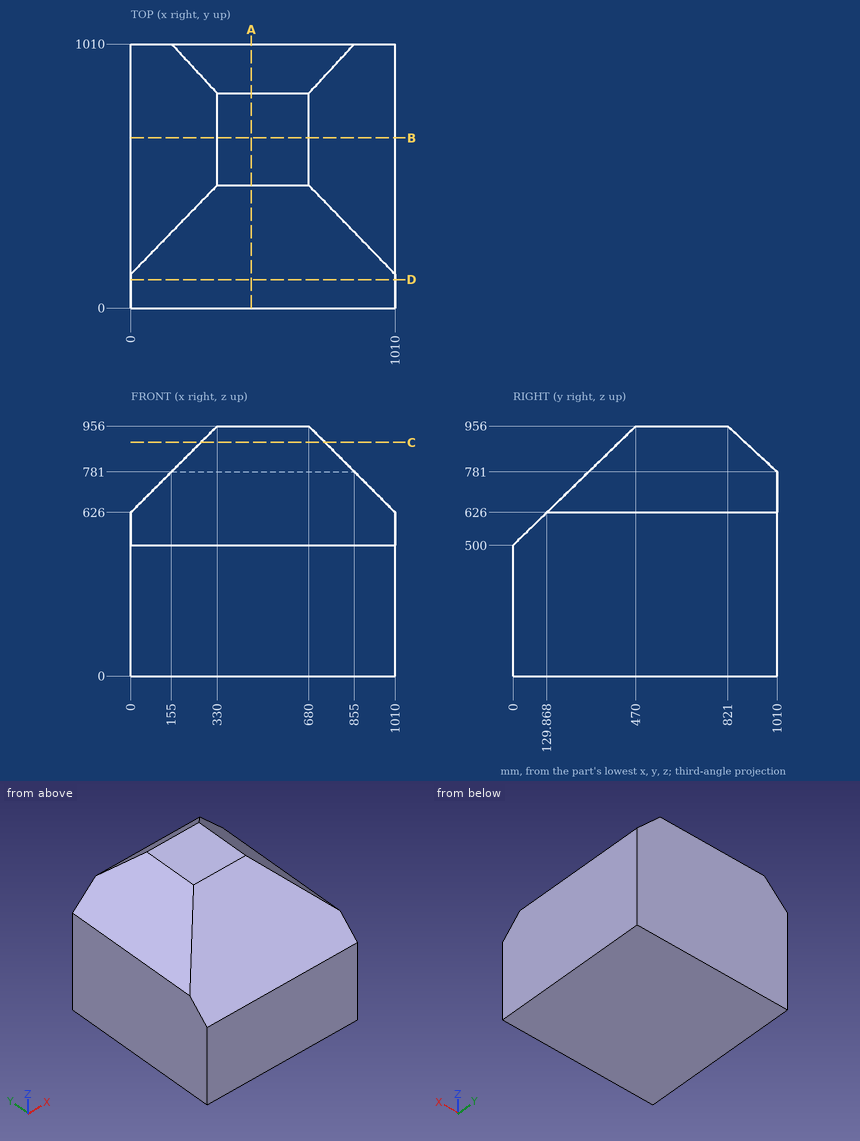
Study the drawing (mm; zero at the part's minimum x, y, z) and answer. Coordinates: 2 decimals unless noted, no trailing zeros. Write each loop counter-clockwise with the first axis right and the second up, starting at its lowest first coordinate (ties: lowest second). Pieces come first, ordered by that corner, then holes.
Q1. Section B-B, the plane y = 650.5 is taken. Write down the section's boundary in (x, z).
Returned:
outline: (0, 0) - (1010, 0) - (1010, 626) - (680, 956) - (330, 956) - (0, 626) - close
Q2. Section A-A, the plane x = 461 is taken. Write down the section's boundary in (y, z).
Returned:
outline: (0, 0) - (1010, 0) - (1010, 781) - (821, 956) - (470, 956) - (0, 500) - close
Q3. Find the intervals of material crossed by line 1 along X through (y, z) = (655.5, 748); line 2 along Z through (x, y) = (707, 577); line 3 along Y through (x, z) = (162, 761.5), in increasing order.
Returned:
line 1: x = 122 to 888
line 2: z = 0 to 929
line 3: y = 269.53 to 1010
Q4. Section C-C, the plane z = 893.5 is taken. Write down the section's boundary in (x, y).
Returned:
outline: (267.5, 405.58) - (742.5, 405.58) - (742.5, 888.5) - (267.5, 888.5) - close
Q5. Given P1, Ø5, axis at x = 594, z = 720, coming from the -Y side; P2, Ø6, axis at y = 765.5, z = 637.5, coming from the -X side, each flat-ended and moving along its own axis, determine where each tip first touches the part or whether it passes through.
Returned:
P1: stops at y = 224.18
P2: stops at x = 8.5
Q6. Section D-D, the plane y = 109 is taken. Write down the section's boundary in (x, z).
Returned:
outline: (0, 0) - (1010, 0) - (1010, 605.75) - (0, 605.75) - close
